Design review of the part shown in the three views and the two pictorial views. Dimensions are in mm from the part's minimum x, y and z. Round coordinates to 2 decimals unless told otherwise and drop trailing zeros. Loops run counter-clockwise (first coordinate to the right, second up) from the corner with the lowest first, then second, coordinate; pieces in that order, holes last. Notation, with made-up numbers: (28, 56) -> (36, 56) arc R20 cw to (36, 73) -> close; hole circle Ø4 at (-16, 15.5). An arc over 180 degrees is marked (long way). One line per question, with ' | ' between items. Start each with the question number.
1. Consider section C-C (x = 0.35). Write out the cut boundary in (y, z), and give its area (3 significant figures).
2. Consider section D-D (x = 1). Write out the cut boundary in (y, z), and give its area (3 significant figures).
3. Draft analysis for pull direction Z (two halves, no side actions). For the marked faces 1, 2 and 3, state which applies: pulls with the +Z half, pulls with the -Z half, needs draft (parallel to the pull), parting line crosses it, or undercut.
4. Wall thickness on line 1 along X through (y, z) = (8.5, 8.25); line 2 along Y through (x, z) = (0.75, 5.15): over which ranges is each line inside the solid? List them lowest first.
5. For pin 1 Ø5 at (y, z) = (4, 5) entering from +X, flat-tipped, find the tip position at first contact; note if it passes through.
6. Consider section A-A (y = 5.15). Write out the cut boundary in (x, z).
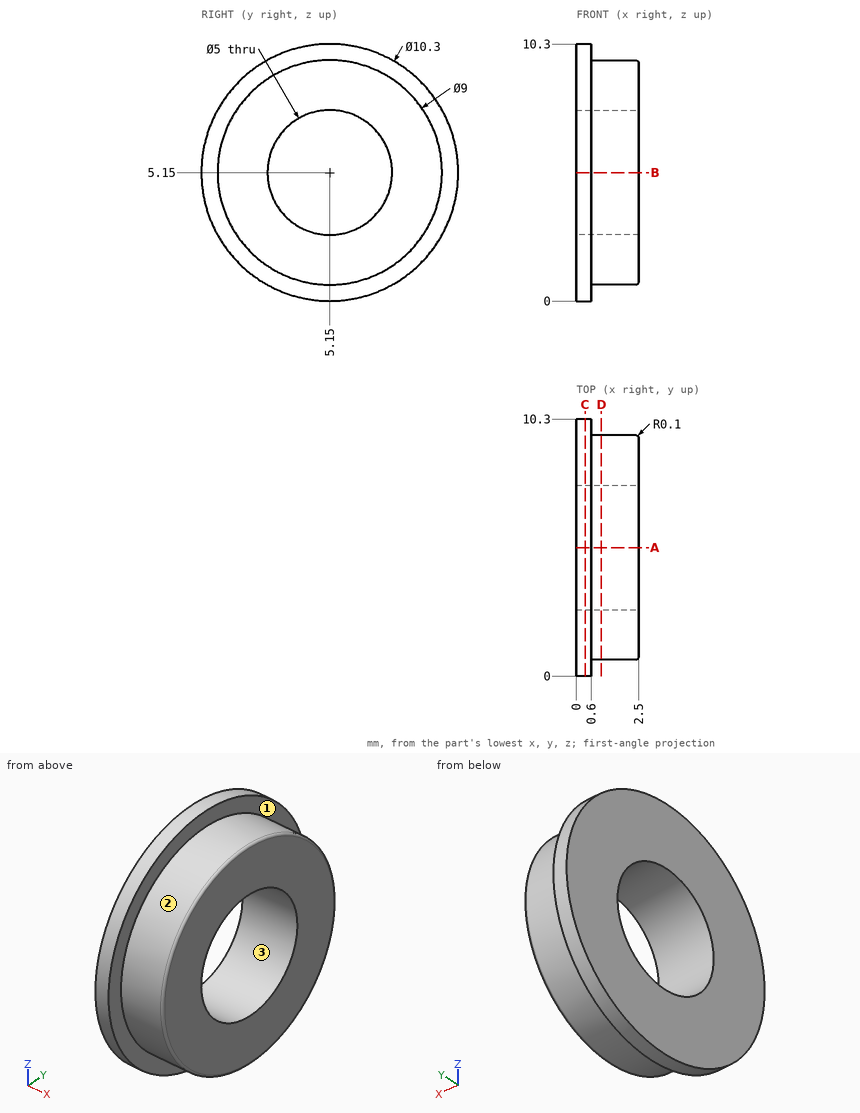
Answer block:
1) outline: circle Ø10.3 at (5.15, 5.15); hole circle Ø5 at (5.15, 5.15) | area: 63.7 mm2
2) outline: circle Ø9 at (5.15, 5.15); hole circle Ø5 at (5.15, 5.15) | area: 44.0 mm2
3) face 1: needs draft | face 2: parting line crosses it | face 3: undercut
4) line 1: x = 0 to 0.6 | line 2: y = 0.65 to 2.65, 7.65 to 9.65
5) pin 1: stops at x = 2.5
6) outline: (0, 0) -> (0.6, 0) -> (0.6, 0.65) -> (2.4, 0.65) arc R0.1 ccw to (2.5, 0.75) -> (2.5, 2.65) -> (0, 2.65) -> close; (0, 7.65) -> (2.5, 7.65) -> (2.5, 9.55) arc R0.1 ccw to (2.4, 9.65) -> (0.6, 9.65) -> (0.6, 10.3) -> (0, 10.3) -> close
